Here's how the part is built. I have some questions about the finished solid (model axes, mm). A direction names the side the tool comes from. Coordinates: 2 decimals unless noted, no trailing zeros. Write each loop counter-clockwise with the first axis right and the second up, starting at its lowest first coordinate (ties: lowest second). Pieces come first, ordered by that corner, then holes. Notation, with made-up numbers: (55, 85) -> (87, 85) arc R20 cw to (87, 123) -> close; hole circle Ø10 at (1, -15.75). An arc over 180 degrees is marked (long way). Put each result on its own line as item: value.
```python
from build123d import *

# Parameters (mm, degrees)
SKETCH1_W           = 30
SKETCH1_H           = 15
BOSS_EXTRUDE1_DEPTH = 2
SKETCH2_W           = 19
SKETCH2_H           = 15
BOSS_EXTRUDE2_DEPTH = 2
SKETCH3_R           = 1.5
CUT_EXTRUDE1_DEPTH  = 2
FILLET1_R           = 3
SKETCH4_W           = 2
SKETCH4_H           = 4
BOSS_EXTRUDE3_DEPTH = 2


with BuildPart() as part:
    # Sketch1 → Boss-Extrude1 (new body)
    with BuildSketch(Plane.XY):
        with Locations((15, 7.5)):
            Rectangle(SKETCH1_W, SKETCH1_H)
    extrude(amount=BOSS_EXTRUDE1_DEPTH)

    # Sketch2 → Boss-Extrude2 (add)
    with BuildSketch(Plane(origin=(30, 0, 0), x_dir=(0, 0, -1), z_dir=(1, 0, 0))):
        with Locations((7.5, 7.5)):
            Rectangle(SKETCH2_W, SKETCH2_H)
    extrude(amount=BOSS_EXTRUDE2_DEPTH)

    # Sketch3 → Cut-Extrude1 (cut)
    with BuildSketch(Plane(origin=(32, 0, 0), x_dir=(0, 0, -1), z_dir=(1, 0, 0))):
        with Locations((10.5, 7.5)):
            Circle(SKETCH3_R)
    extrude(amount=-CUT_EXTRUDE1_DEPTH, mode=Mode.SUBTRACT)

    # Fillet1
    fillet1_edges = [part.edges().sort_by_distance(p)[0] for p in [
        (31, 0, -17),
        (31, 15, -17),
    ]]
    fillet(fillet1_edges, radius=FILLET1_R)

    # Sketch4 → Boss-Extrude3 (add)
    with BuildSketch(Plane.ZY):
        with Locations((1, 13)):
            Rectangle(SKETCH4_W, SKETCH4_H)
        with Locations((1, 2)):
            Rectangle(SKETCH4_W, SKETCH4_H)
    extrude(amount=BOSS_EXTRUDE3_DEPTH)


solid = part.part
```
Item 1: Imagine slicing it at B-B on z = -10.5. Write out the boundary of the cut face in (x, y), then the cut area to 3 significant figures.
Output:
outline: (30, 0) -> (32, 0) -> (32, 6) -> (30, 6) -> close; (30, 9) -> (32, 9) -> (32, 15) -> (30, 15) -> close
area: 24.0 mm²
Item 2: If we mould it in two halves opening along Z, with no side actions, what happens to faces 1 (the cylindrical face through (31.014, 6.036, -10.175)), 2 (the flat face through (32, 8, -7)), 3 (the flat face through (14, 7, 0))? For each: released by +Z, released by -Z, zero draft, split by the parting line, or undercut.
Output:
face 1: undercut
face 2: zero draft
face 3: released by -Z
Item 3: For P1, Ø1, axis at y = 8.5, z = 1, coming from the -X side; P2, Ø1.5, axis at y = 8.5, z = -8.5, coming from the -X side; P3, Ø1, axis at x = 10.5, y = 7, coming from the -Z side; P4, Ø1.5, axis at x = 28, z = -12.5, coming from the +Y side, each with a flat end and sliding along its axis, tell me the tip position at first contact or that it passes through.
Output:
P1: stops at x = 0
P2: stops at x = 30
P3: stops at z = 0
P4: passes through
Item 4: Imagine slicing it at A-A on y = 7.5. Write out the boundary of the cut face in (x, z), then the cut area to 3 significant figures.
Output:
outline: (0, 0) -> (30, 0) -> (30, -9) -> (32, -9) -> (32, 2) -> (0, 2) -> close; (30, -17) -> (32, -17) -> (32, -12) -> (30, -12) -> close
area: 92.0 mm²
Item 5: Imagine slicing it at D-D on z = -7.25. Write out the boundary of the cut face in (x, y).
Output:
outline: (30, 0) -> (32, 0) -> (32, 15) -> (30, 15) -> close
Item 6: Please list where these lines run through material, in increasing order: line 1 along Y through (x, z) = (31.15, -10.5); line 2 along X through (y, z) = (5.75, -6.25); line 3 along Z through (x, y) = (17, 5.25). Write a range as from..to.
Output:
line 1: y = 0..6, 9..15
line 2: x = 30..32
line 3: z = 0..2
Item 7: Imagine slicing it at C-C on x = 13.5. Write out the boundary of the cut face in (y, z), then the cut area to 3 significant figures.
Output:
outline: (0, 0) -> (15, 0) -> (15, 2) -> (0, 2) -> close
area: 30.0 mm²
Item 8: Which directions (+Z, -Z, +X, -X, +Y, -Y) give clear straight access to the entire face, cutting with the end or side of a thin tool? Please do faces 4 (the flat face through (30, 8, -8)), 5 (the flat face through (-1, 11, 1)), 6 (the flat face through (-2, 13, 1)).
Output:
face 4: -Z, -X, +Y, -Y
face 5: +Z, -Z, -X
face 6: +Z, -Z, -X, +Y, -Y
